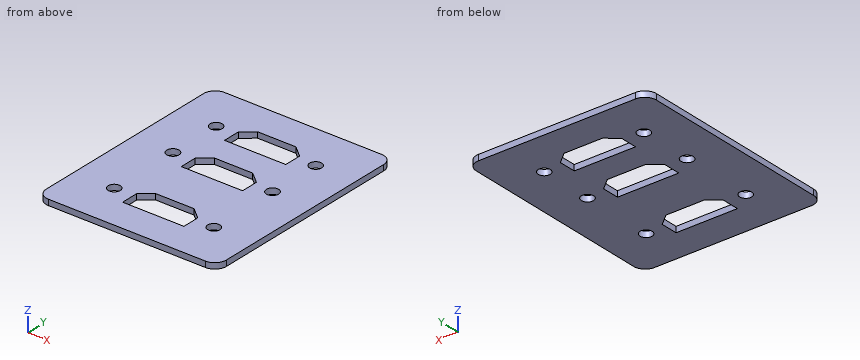
from build123d import *

# Parameters (mm, degrees)
F0_R     = 1.6
F1_DEPTH = 1.5


with BuildPart() as f1:
    # F0 (on Top) → F1 (new body)
    with BuildSketch(Plane.XY):
        with BuildLine():
            Line((-20.5, -31), (20.5, -31))
            ThreePointArc((20.5, -31), (22.62132, -30.12132), (23.5, -28))
            Line((23.5, -28), (23.5, 23))
            ThreePointArc((23.5, 23), (22.62132, 25.12132), (20.5, 26))
            Line((20.5, 26), (-20.5, 26))
            ThreePointArc((-20.5, 26), (-22.62132, 25.12132), (-23.5, 23))
            Line((-23.5, 23), (-23.5, -28))
            ThreePointArc((-23.5, -28), (-22.62132, -30.12132), (-20.5, -31))
        make_face()
        with Locations((-13, -19)):
            Circle(F0_R, mode=Mode.SUBTRACT)
        Polygon((-8, -18), (-5, -15.5), (5, -15.5), (8, -18), (8, -22.5), (-8, -22.5), align=None, mode=Mode.SUBTRACT)
        with Locations((13, -19)):
            Circle(F0_R, mode=Mode.SUBTRACT)
        with Locations((-13, 0)):
            Circle(F0_R, mode=Mode.SUBTRACT)
        with Locations((-13, 14)):
            Circle(F0_R, mode=Mode.SUBTRACT)
        Polygon((-8, 1), (-5, 3.5), (5, 3.5), (8, 1), (8, -3.5), (-8, -3.5), align=None, mode=Mode.SUBTRACT)
        with Locations((13, 0)):
            Circle(F0_R, mode=Mode.SUBTRACT)
        Polygon((-8, 15), (-5, 17.5), (5, 17.5), (8, 15), (8, 10.5), (-8, 10.5), align=None, mode=Mode.SUBTRACT)
        with Locations((13, 14)):
            Circle(F0_R, mode=Mode.SUBTRACT)
    extrude(amount=F1_DEPTH)


solid = f1.part
Design review of the part built by this model. Coordinates are the model's own, in mm. Coordinates: 2 decimals unless noted, no trailing zeros. Loops run counter-clockwise (first coordinate to the right, second up) from the corner with the lowest first, then second, coordinate; pieces in that order, holes last. Notation, with made-up numbers: M 73.25,-36.75 L 100.25,-36.75 A32 cw 100.25,-5.75 Z; hole C 51.25,-31 d7. An arc over 180 degrees is marked long. Use one line per item in the form item = value.
(1) Consider section B-B (x = -13). Write out the cut boundary in (y, z), and give its area (3 significant figures).
Return value:
outline = M -31,0 L -20.6,0 L -20.6,1.5 L -31,1.5 Z; M -17.4,0 L -1.6,0 L -1.6,1.5 L -17.4,1.5 Z; M 1.6,0 L 12.4,0 L 12.4,1.5 L 1.6,1.5 Z; M 15.6,0 L 26,0 L 26,1.5 L 15.6,1.5 Z
area = 71.1 mm2
(2) Consider section C-C (y = -19). Write out the cut boundary in (x, z), and give its area (3 significant figures).
Return value:
outline = M -23.5,0 L -14.6,0 L -14.6,1.5 L -23.5,1.5 Z; M -11.4,0 L -8,0 L -8,1.5 L -11.4,1.5 Z; M 8,0 L 11.4,0 L 11.4,1.5 L 8,1.5 Z; M 14.6,0 L 23.5,0 L 23.5,1.5 L 14.6,1.5 Z
area = 36.9 mm2
(3) For line 1 along Y through (x, z) = (-13, 0.6); line 2 along Y through (x, z) = (4, 1.1); line 3 along X through (y, z) = (14.5, 0.2), list the stretches that pass through material, from the lowest coordinate up. Write a range as from..to.
Return value:
line_1 = -31..-20.6, -17.4..-1.6, 1.6..12.4, 15.6..26
line_2 = -31..-22.5, -15.5..-3.5, 3.5..10.5, 17.5..26
line_3 = -23.5..-14.52, -11.48..-8, 8..11.48, 14.52..23.5
(4) Clearance check with a flat-ended pin moving along its axis: P1, Ø1.9, axis at x = 13, y = 14, coming from the -Z side. State where the tip first meets the part, or that it passes through.
Return value:
P1 = through
(5) Consider section A-A (z = 1.25). Give the number of separate pieces and of enclosed holes in the cut face, and give its area (3 significant figures).
Return value:
separate_pieces = 1
enclosed_holes = 9
area = 2,310 mm2
